Input: part model. Units: mm. Frame: model coordinates. A direction names the side the tool comes from. Give positions to 0.01 mm unless a question says otherwise; leave off trailing zeros. Order: outer loops, then holes, each group sorted by start corner. A loop starts at its lowest first (then second) coordinate and runs counter-clockwise, first axis right, second up. Notation, with made-up numbers: (-34.5, 37) - (2.5, 37) arc R18 cw to (2.5, 69) - close; hole circle Ø1 at (51.5, 43). An arc over 180 degrees is marked (long way). Use a Markdown table: item, result.
from build123d import *

# Parameters (mm, degrees)
SCHIZZO2_R               = 20
TAGLIO_ESTRUSIONE1_DEPTH = 184.962632075
SMUSSO1_SIZE             = 2
RACCORDO1_R              = 1
TAGLIO_ESTRUSIONE2_START = -35
TAGLIO_ESTRUSIONE2_DEPTH = 5


with BuildPart() as part:
    # Schizzo1 → Rivoluzione1 (revolve)
    with BuildSketch(Plane.XY, mode=Mode.PRIVATE) as rivoluzione1_sk:
        Polygon((0, 0), (0, 27.5), (17, 27.5), (17, 26), (19, 26), (19.866025404, 27.5), (40, 27.5), (40, 35), (109.5, 35), (109.5, 39), (115.5, 39), (115.5, 35), (140.5, 35), (140.5, 32.5), (152.633974596, 32.5), (153.5, 31), (156, 31), (156, 32.5), (175.5, 32.5), (175.5, 0), align=None)
    revolve(rivoluzione1_sk.sketch.rotate(Axis((0, 0, 0), (1, 0, 0)), 90), axis=Axis((0, 0, 0), (1, 0, 0)))

    # Schizzo2 → Taglio-Estrusione1 (cut, through all)
    with BuildSketch(Plane.ZY):
        with BuildLine():
            ThreePointArc((-6, 19.078784028), (-3.035153986, 19.768354516), (0, 20))
            Line((0, 20), (0, 23.3))
            Line((0, 23.3), (-6, 23.3))
            Line((-6, 23.3), (-6, 19.078784028))
        make_face()
        with BuildLine():
            Line((0, 23.3), (0, 20))
            ThreePointArc((0, 20), (3.035153986, 19.768354516), (6, 19.078784028))
            Line((6, 19.078784028), (6, 23.3))
            Line((6, 23.3), (0, 23.3))
        make_face()
        Circle(SCHIZZO2_R)
    extrude(amount=-TAGLIO_ESTRUSIONE1_DEPTH, mode=Mode.SUBTRACT)

    # Smusso1
    smusso1_edges = [part.edges().sort_by_distance(p)[0] for p in [
        (175.5, 0, -32.5),
        (40, 0, -35),
        (0, 0, -27.5),
    ]]
    chamfer(smusso1_edges, length=SMUSSO1_SIZE)

    # Raccordo1
    raccordo1_edges = [part.edges().sort_by_distance(p)[0] for p in [
        (140.5, 0, -32.5),
        (115.5, 0, -35),
        (109.5, 0, -35),
    ]]
    fillet(raccordo1_edges, radius=RACCORDO1_R)

    # Schizzo3 → Taglia-Rivoluzione1 (revolve, cut)
    with BuildSketch(Plane.XY, mode=Mode.PRIVATE) as taglia_rivoluzione1_sk:
        Polygon((48.366025404, 35), (47.5, 33.5), (44.85, 33.5), (44.85, 35), align=None)
    revolve(taglia_rivoluzione1_sk.sketch.rotate(Axis((-16.412152114, 0, 0), (1, 0, 0)), 90), axis=Axis((-16.412152114, 0, 0), (1, 0, 0)), mode=Mode.SUBTRACT)

    # Schizzo4 → Taglio-Estrusione2 (cut)
    with BuildSketch(Plane(origin=(0, 0, 0), x_dir=(1, 0, 0), z_dir=(0, 1, 0)).offset(TAGLIO_ESTRUSIONE2_START)):
        with BuildLine():
            Line((60.5, 10), (96.5, 10))
            ThreePointArc((96.5, 10), (106.5, 0), (96.5, -10))
            Line((96.5, -10), (60.5, -10))
            ThreePointArc((60.5, -10), (50.5, 0), (60.5, 10))
        make_face()
    extrude(amount=TAGLIO_ESTRUSIONE2_DEPTH, mode=Mode.SUBTRACT)


solid = part.part
1. Pin query (flat end, axial travel): pin 1 (4.5 mm diameter, centred on x = 104.5, y = 22, fed in from +Z); pin 2 (5 mm diameter, centred on x = 34.5, z = 3.5, fed in from -Y); pin 3 (1.3 mm diameter, centred on x = 98.5, y = 22, fed in from -Z); pin 4 (3 mm diameter, centred on y = 13, z = -13, fed in from +X). Return the tip coordinate at first contact, or that it passes through.
Response:
| item | result |
|---|---|
| pin 1 | stops at z = 28.9 |
| pin 2 | stops at y = -27.48 |
| pin 3 | stops at z = -27.73 |
| pin 4 | passes through |
2. Set-up query: faces 4 (the face through (40, -25, 12)), 5 (the face through (128.668, 34.168, -7.587)), 6 (the face through (87, 23.3, 0)), 7 (the face through (46.2, 29.7, 15.5)), 8 (the face through (50.5, -32, 0.2)). Return all of +Z, -Z, +X, -X, +Y, -Y with unobstructed straight access to the full face (end or side cutting, diameter ignored); none if empty.
Response:
| item | result |
|---|---|
| face 4 | -X |
| face 5 | +X |
| face 6 | +X, -X |
| face 7 | none |
| face 8 | -Y |
3. Section query B-B (x = 13.5). Return loops of the section in (y, z), then the cut area to 3 significant figures.
Response:
| item | result |
|---|---|
| outline | circle Ø55 at (0, 0); hole (19.08, -6) - (23.3, -6) - (23.3, 6) - (19.08, 6) arc R20 ccw (long way) to start |
| area | 1,080 mm^2 |
4. Section query A-A (x = 65.5). Return loops of the section in (y, z).
Response:
| item | result |
|---|---|
| outline | (-33.54, -10) arc R35 ccw (long way) to (-33.54, 10) - (-30, 10) - (-30, -10) - close; hole (19.08, -6) - (23.3, -6) - (23.3, 6) - (19.08, 6) arc R20 ccw (long way) to start |
5. Material intervals for line 1 along Y through (x, z) = (15, 0.5); line 2 along Z through (x, y) = (96.5, -18.5); line 3 along Z through (x, y) = (88.5, 13.5), sorted ascending.
Response:
| item | result |
|---|---|
| line 1 | y = -27.5 to -19.99, 23.3 to 27.5 |
| line 2 | z = -29.71 to -7.6, 7.6 to 29.71 |
| line 3 | z = -32.29 to -14.76, 14.76 to 32.29 |
6. Mould query, pull axis Y, two halves, no side actions, for faces 1 (the face through (164.87, -9.76, 31)), 2 (the face through (156, 12, -29)), 3 (the face through (86.522, -19.984, -0.794)). Classes: pulls with the +Y half, pulls with the -Y half, needs draft (parallel to the pull), parting line crosses it, or undercut.
Response:
| item | result |
|---|---|
| face 1 | parting line crosses it |
| face 2 | needs draft |
| face 3 | undercut |
7. Section query C-C (x = 137). Return loops of the section in (y, z).
Response:
| item | result |
|---|---|
| outline | circle Ø70 at (0, 0); hole (19.08, -6) - (23.3, -6) - (23.3, 6) - (19.08, 6) arc R20 ccw (long way) to start |
